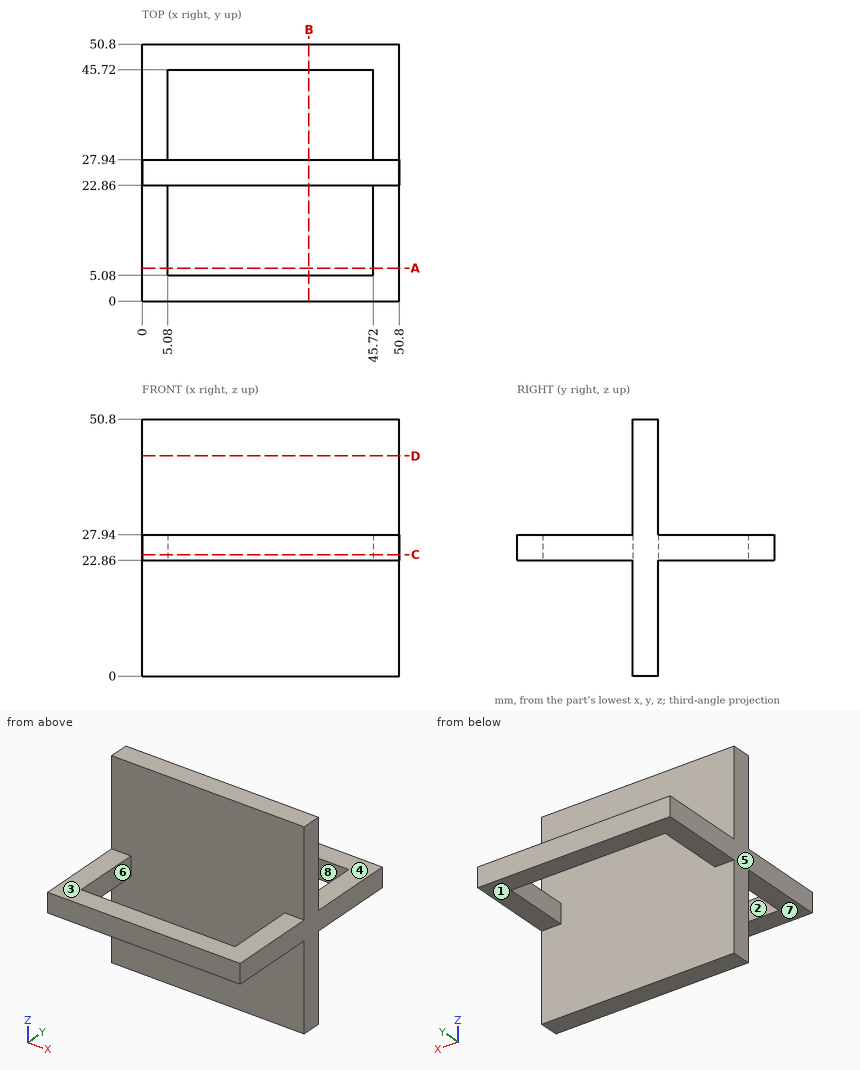
Source: three-view drawing plus pictorial views. Frame: mm from the lowest corner of the part. A direction names the side the tool comes from. Coordinates: 2 decimals unless noted, no trailing zeros. Order: outer loops, then holes, each group sorted by start corner. A loop starts at its lowest first (then second) coordinate and runs counter-clockwise, first axis right, second up. Notation, with made-up numbers: M 46,-28 L 89,-28 A29 ccw 89,-7 Z; hole C 48.5,-9 d10. An arc over 180 degrees is marked long. Answer in a Markdown table with one row per item.
(1) Section query D-D, the plane z = 43.5. Output: boundary loops of the cut face in (x, y), plus the area to 3 significant figures.
Numbers:
| item | result |
|---|---|
| outline | M 0,22.86 L 50.8,22.86 L 50.8,27.94 L 0,27.94 Z |
| area | 258 mm^2 |
(2) Draft query along X for the marked faces 5, 6, 7 and 8. Return one class per face: pulls with the +X half, pulls with the -X half, needs draft (parallel to the pull), parting line crosses it, or undercut.
Numbers:
| item | result |
|---|---|
| face 5 | pulls with the -X half |
| face 6 | undercut |
| face 7 | needs draft |
| face 8 | undercut |
(3) Section query C-C, the plane z = 24. Output: boundary loops of the cut face in (x, y).
Numbers:
| item | result |
|---|---|
| outline | M 0,0 L 50.8,0 L 50.8,50.8 L 0,50.8 Z; hole M 5.08,5.08 L 45.72,5.08 L 45.72,22.86 L 5.08,22.86 Z; hole M 5.08,27.94 L 45.72,27.94 L 45.72,45.72 L 5.08,45.72 Z |
(4) Access query for the marked faces 1, 2, 3 and 4. Directions: +Z, -Z, +X, -X, +Y, -Y. A direction counts if a zero-diameter tool reaches every point of the face in a straight line with its end or side. Return the directions, or none.
Numbers:
| item | result |
|---|---|
| face 1 | -Z, +X, -X, +Y |
| face 2 | +Z, -Z |
| face 3 | +Z, +X, -X, -Y |
| face 4 | +Z, +X, -X, +Y |
(5) Material intervals for line 1 (Y direction, x = 33, z = 26.5); line 2 (Y direction, x = 46.5, z = 19.5), sorted ascending. Write a range as [from, to].
Numbers:
| item | result |
|---|---|
| line 1 | y = [0, 5.08], [22.86, 27.94], [45.72, 50.8] |
| line 2 | y = [22.86, 27.94] |
(6) Section query A-A, the plane y = 6.5. Output: boundary loops of the cut face in (x, z).
Numbers:
| item | result |
|---|---|
| outline | M 0,22.86 L 5.08,22.86 L 5.08,27.94 L 0,27.94 Z; M 45.72,22.86 L 50.8,22.86 L 50.8,27.94 L 45.72,27.94 Z |
(7) Contact query for flat-ended pins moving along their axis: pin 1 Ø3 at (x, z) = (33.5, 15.5) entering from +Y; pin 2 Ø11.5 at (x, y) = (25.5, 41) entering from -Z; pin 3 Ø5 at (x, z) = (25.5, 35.5) entering from -Y; pin 4 Ø10 at (x, y) = (27.5, 34) entering from -Z. Output: stop coordinate, or through.
Numbers:
| item | result |
|---|---|
| pin 1 | stops at y = 27.94 |
| pin 2 | stops at z = 22.86 |
| pin 3 | stops at y = 22.86 |
| pin 4 | passes through |
(8) Section query B-B, the plane x = 33. Output: boundary loops of the cut face in (y, z).
Numbers:
| item | result |
|---|---|
| outline | M 0,22.86 L 5.08,22.86 L 5.08,27.94 L 0,27.94 Z; M 22.86,0 L 27.94,0 L 27.94,50.8 L 22.86,50.8 Z; M 45.72,22.86 L 50.8,22.86 L 50.8,27.94 L 45.72,27.94 Z |
